Input: part model. Units: mm. Frame: model coordinates. A direction names the side the tool comes from. Coordinates: 2 decimals unless noted, no trailing zeros. Order: outer loops, then holes, each group sorted by start corner. A loop starts at its lowest first (then second) coordinate and runs counter-clockwise, first axis right, second up.
Autodesk Inventor part; units mm, degrees
ref_plane "YZ Plane" through (0, 0, 0) normal (1, 0, 0) x (0, 1, 0)
ref_plane "XZ Plane" through (0, 0, 0) normal (0, 1, 0) x (-1, 0, 0)
ref_plane "XY Plane" through (0, 0, 0) normal (0, 0, 1) x (1, 0, 0)
sketch "Sketch3" plane through (0, 0, 0) normal (1, 0, 0) x (0, 1, 0)
  line L0 (-27.1198, 0) -> (-27.1198, -16.51)
  line L1 (27.1198, 0) -> (27.1198, -16.51)
  arc A0 (-27.1198, -16.51) -> (27.1198, -16.51) centre (0, 0) ccw
  line L2 (27.1198, 0) -> (-27.1198, 0)
revolve "Revolution2" add sketch "Sketch3" angle 360 about axis through (0, 27.1198, 0) along (0, -1, 0)
sketch "Sketch5" plane through (0, 27.1198, 0) normal (0, 1, 0) x (1, 0, 0)
  circle A0 centre (0, 0) radius 1.5875
  dimension "d7" = 3.175
extrude "Extrusion1" cut sketch "Sketch5" against normal blind 23.6728
sketch "Sketch6" plane through (0, 0, 0) normal (1, 0, 0) x (0, 1, 0)
  line L0 (27.1198, 16.51) -> (27.1198, -16.51)
  line L1 (27.1198, 16.51) -> (54.2396, 0)
  line L2 (54.2396, 0) -> (27.1198, -16.51)
  line L3 (27.1198, 16.51) -> (27.1198, -16.51)
  arc A0 (22.4896, 0) -> (27.1198, -16.51) centre (54.2396, 0) ccw
  line L4 (85.9896, 0) -> (22.4896, 0)
  point P0 (0, 0)
  point P1 (27.1198, 0)
  dimension "d10" = 31.75
  dimension "d11" = 31.75
  dimension "d12" = 33.02
  dimension "d13" = 63.5
revolve "Revolution3" cut sketch "Sketch6" angle 360 about axis through (0, 85.9896, 0) along (0, -1, 0) contours L0 A0 L4
sketch "Sketch7" plane through (0, -27.1198, 0) normal (0, -1, 0) x (1, 0, 0)
  circle A0 centre (0, 0) radius 1.5875
  circle A1 centre (0, 0) radius 1.5875
  point P0 (0, 0)
extrude "Extrusion2" cut sketch "Sketch7" against normal blind 23.6728
sketch "Sketch8" plane through (0, 0, 0) normal (1, 0, 0) x (0, 1, 0)
  line L0 (-27.1198, 16.51) -> (-27.1198, -16.51)
  line L1 (-27.1198, 16.51) -> (-27.1198, -16.51)
  line L2 (-27.1198, -16.51) -> (-54.2396, 0)
  line L3 (-54.2396, 0) -> (-27.1198, 16.51)
  circle A0 centre (-54.2396, 0) radius 31.75
  line L4 (-54.2396, 0) -> (-22.4896, 0)
  point P0 (0, 0)
  point P1 (-27.1198, 0)
  point P2 (-22.4896, 0)
  dimension "d17" = 33.02
  dimension "d18" = 31.75
  dimension "d19" = 31.75
  dimension "d20" = 31.75
revolve "Revolution4" cut sketch "Sketch8" angle 360 about axis through (0, -54.2396, 0) along (0, 1, 0) picked at (-26.272, 9.2768) contours A0 L4 L0
sketch "Sketch9" plane through (0, 0, 0) normal (0, 1, 0) x (-1, 0, 0)
  circle A0 centre (0, 0) radius 31.75
  line L0 (30.7725, 7.8175) -> (7.1862, 30.9261)
  line L1 (-30.7725, 7.8175) -> (-7.1862, 30.9261)
extrude "Extrusion3" cut sketch "Sketch9" along normal mid plane 101.6 contours A0 L1 L0 keep common part
sketch "Sketch10" plane through (18.9794, 0, 19.3718) normal (0.6998, 0, 0.7143) x (0.7143, 0, -0.6998)
  circle A0 centre (0, 0) radius 1.5875
  dimension "d24" = 3.175
extrude "Extrusion4" add sketch "Sketch10" along normal blind 23.6728
sketch "Sketch11" plane through (-18.9794, 0, 19.3718) normal (-0.6998, 0, 0.7143) x (0.7143, 0, 0.6998)
  circle A0 centre (0, 0) radius 1.5875
  dimension "d27" = 3.175
extrude "Extrusion5" add sketch "Sketch11" along normal blind 23.6728
sketch "Sketch12" plane through (0, 0, 0) normal (0, 1, 0) x (-1, 0, 0)
  circle A0 centre (0, 0) radius 1.5875
  circle A1 centre (0, 0) radius 31.75
  arc A2 (-30.7725, 7.8175) -> (-7.1862, 30.9261) centre (0, 0) ccw
  line L0 (-31.75, 0) -> (31.75, 0)
  point P0 (-1.5875, 0)
  point P1 (1.5875, 0)
  point P2 (31.75, 0)
revolve "Revolution5" add sketch "Sketch12" angle 110 mid plane about axis through (31.75, 0, 0) along (-1, 0, 0) picked at (21.4293, 2.3601) contours A0 L0 A1
properties part number "solid mid ball"
Item 1: Cut plane C-C on x = 17.5. Return loops of the section in (y, z), then the cut area to 3 significant figures.
Response values:
outline: (-0.03, -26.49) - (0.03, -26.49) arc R26.49 ccw (long way) to start
area: 2,200 mm2
Item 2: Ray query, probe 1 along Z at (x, y) = (0, -9.25); probe 2 along X at (y, z) = (-12, 1); probe 3 along Z at (x, y) = (18, 4.5). Return the intervals inside material, ascending.
Response values:
probe 1: z = -30.37 to -1.59, 1.59 to 30.37
probe 2: x = -29.38 to -1.23, 1.23 to 29.38
probe 3: z = -25.76 to 25.76
Item 3: Draft query along X for faces 4 (the face through (35.53, 0.02, 36.3)), 5 (the face through (-35.56, 0.02, 36.27)), 6 (the face through (27.64, -0.07, 30.48)). Return one class per face: pulls with the +X half, pulls with the -X half, needs draft (parallel to the pull), parting line crosses it, or undercut.
Response values:
face 4: pulls with the +X half
face 5: pulls with the -X half
face 6: undercut
Item 4: Cut plane B-B on z = -23. Return loops of the section in (x, y).
Response values:
outline: (-21.89, -0.03) arc R21.89 ccw to (21.89, -0.03) - (21.89, 0.03) arc R21.89 ccw to (-21.89, 0.03) - close
Item 5: Cut plane D-D on y = 6. Return loops of the section in (x, z) (1 decimal).
Response values:
outline: circle Ø62.4 at (0, 0); hole circle Ø3.2 at (0, 0)
Item 6: Cut plane A-A on y = 18. Return loops of the section in (x, z) (1 decimal).
Response values:
outline: circle Ø52.3 at (0, 0); hole circle Ø3.2 at (0, 0)
Item 7: Access query for faces 1 (the face through (0, -3.447, 0)), 2 (the face through (-29.675, 0.966, 28.489)), 3 (the face through (-0.34, 13.12, 1.55)). Directions: +Z, -Z, +X, -X, +Y, -Y. A direction counts if a zero-diameter tool reaches every point of the face in a straight line with its end or side. Return the directions, or none.
Response values:
face 1: -Y
face 2: none
face 3: +Y
Item 8: Pin query (flat end, axial travel): pin 1 Ø1.5 at (x, z) = (-4.5, -17.5) entering from -Y; pin 2 Ø1 at (x, z) = (0, -0.5) entering from +Y; pin 3 Ø8 at (x, y) = (3.5, -17) entering from -Z; pin 4 Ø5 at (x, z) = (-10.5, 12.5) entering from +Y. Return the tip coordinate at first contact, or that it passes through.
Response values:
pin 1: stops at y = -26.61
pin 2: stops at y = 3.45
pin 3: stops at z = -28.8
pin 4: stops at y = 27.12
